Here's how the part is built. I have some questions about the finished solid (model axes, mm). Face numbers are marked on the shaded views. A direction names the side the tool comes from. Give positions to 0.01 mm unless a question says otherwise; leave off trailing zeros. Write each loop counter-clockwise with the first axis right and the second up, starting at its lowest first coordinate (ties: lowest second). Pieces come first, ordered by that corner, then holes. Notation, with made-up numbers: (-38.75, 10.25) - (3.25, 10.25) arc R31 cw to (3.25, 47.25) - close; hole circle Ø4 at (-35.5, 44). An arc over 180 degrees is marked (long way). Use one line per item in the form item = value. Start each with the question number.
from build123d import *

# Parameters (mm, degrees)
SKETCH2_R          = 1.6
CUT_EXTRUDE2_DEPTH = 6
SKETCH4_R          = 1.2
CUT_EXTRUDE4_DEPTH = 5
CHAMFER1_SIZE      = 0.5
CHAMFER3_SIZE      = 0.1


with BuildPart() as part:
    # Sketch1 → Revolve4 (revolve)
    with BuildSketch(Plane.XY, mode=Mode.PRIVATE) as revolve4_sk:
        with BuildLine():
            Line((844.943210176, 281.38888375), (845.428519032, 280.88888375))
            Line((845.428519032, 280.88888375), (849.942387276, 280.88888375))
            Line((849.942387276, 280.88888375), (849.942387276, 290.88888375))
            Line((849.942387276, 290.88888375), (860.942387276, 290.88888375))
            Line((860.942387276, 290.88888375), (860.942387276, 297.88888375))
            Line((860.942387276, 297.88888375), (856.942387276, 297.88888375))
            Line((856.942387276, 297.88888375), (856.942387276, 303.38888375))
            Line((856.942387276, 303.38888375), (853.942387276, 303.38888375))
            Line((853.942387276, 303.38888375), (853.942387276, 302.38888375))
            Line((853.942387276, 302.38888375), (842.942387276, 302.38888375))
            ThreePointArc((842.942387276, 302.38888375), (842.442387276, 302.71356783), (841.942387276, 302.38888375))
            Line((841.942387276, 302.38888375), (840.942387276, 302.38888375))
            Line((840.942387276, 302.38888375), (840.942387276, 299.054998182))
            Line((840.942387276, 299.054998182), (838.850052202, 299.054998182))
            Line((838.850052202, 299.054998182), (838.556543661, 299.38888375))
            Line((838.556543661, 299.38888375), (837.02254839, 299.38888375))
            Line((837.02254839, 299.38888375), (836.904667291, 299.280121777))
            Line((836.904667291, 299.280121777), (836.804319001, 299.38888375))
            Line((836.804319001, 299.38888375), (835.942387276, 299.38888375))
            Line((835.942387276, 299.38888375), (835.942387276, 302.38888375))
            Line((835.942387276, 302.38888375), (834.038239304, 302.38888375))
            Line((834.038239304, 302.38888375), (833.942387276, 302.301556661))
            Line((833.942387276, 302.301556661), (833.862826931, 302.38888375))
            Line((833.862826931, 302.38888375), (831.942387276, 302.38888375))
            Line((831.942387276, 302.38888375), (831.942387276, 261.38888375))
            Line((831.942387276, 261.38888375), (836.942387276, 261.38888375))
            Line((836.942387276, 261.38888375), (836.942387276, 281.38888375))
            Line((836.942387276, 281.38888375), (838.542387276, 281.38888375))
            Line((838.542387276, 281.38888375), (838.791787089, 281.619745582))
            Line((838.791787089, 281.619745582), (843.015951121, 281.619745582))
            Line((843.015951121, 281.619745582), (843.343210176, 281.38888375))
            Line((843.343210176, 281.38888375), (844.943210176, 281.38888375))
        make_face()
    revolve(revolve4_sk.sketch.rotate(Axis((831.942387276, 300.670444461, 0), (0, -1, 0)), 90), axis=Axis((831.942387276, 300.670444461, 0), (0, -1, 0)))

    # Sketch2 → Cut-Extrude2 (cut)
    with BuildSketch(Plane(origin=(0, 302.38888375, 0), x_dir=(-1, 0, 0), z_dir=(0, 1, 0))):
        with Locations(Location((-849.942387276, 0, 0), (0, 0, 90))):
            Circle(SKETCH2_R)
        with Locations(Location((-813.942387276, 0, 0), (0, 0, 90))):
            Circle(SKETCH2_R)
    extrude(amount=-CUT_EXTRUDE2_DEPTH, mode=Mode.SUBTRACT)

    # Cut-Extrude3 cone 1 section (through the dimple's axis) → Cut-Extrude3 (revolve, cut)
    with BuildSketch(Plane(origin=(849.942387276, 296.38888375, 0), x_dir=(0, 0, 1), z_dir=(1, 0, 0))):
        Polygon((0, 0), (1.6, 0), (0, 1.120332061), align=None)
    revolve(axis=Axis((849.942387276, 296.38888375, 0), (0, -1, 0)), mode=Mode.SUBTRACT)

    # Cut-Extrude3 cone 2 section (through the dimple's axis) → Cut-Extrude3 cone 2 (revolve, cut)
    with BuildSketch(Plane(origin=(813.942387276, 296.38888375, 0), x_dir=(0, 0, 1), z_dir=(1, 0, 0))):
        Polygon((0, 0), (1.6, 0), (0, 1.120332061), align=None)
    revolve(axis=Axis((813.942387276, 296.38888375, 0), (0, -1, 0)), mode=Mode.SUBTRACT)

    # Sketch4 → Cut-Extrude4 (cut)
    with BuildSketch(Plane.XZ.offset(-290.88888375)):
        with Locations(Location((831.942387276, -24, 0), (0, 0, 270))):
            Circle(SKETCH4_R)
        with Locations(Location((811.157777585, 12, 0), (0, 0, 270))):
            Circle(SKETCH4_R)
        with Locations(Location((852.726996967, 12, 0), (0, 0, 270))):
            Circle(SKETCH4_R)
    extrude(amount=-CUT_EXTRUDE4_DEPTH, mode=Mode.SUBTRACT)

    # Cut-Extrude5 cone 1 section (through the dimple's axis) → Cut-Extrude5 (revolve, cut)
    with BuildSketch(Plane(origin=(831.942387276, 295.88888375, -24), x_dir=(0, 0, -1), z_dir=(1, 0, 0))):
        Polygon((0, 0), (1.2, 0), (0, 0.840249046), align=None)
    revolve(axis=Axis((831.942387276, 295.88888375, -24), (0, 1, 0)), mode=Mode.SUBTRACT)

    # Cut-Extrude5 cone 2 section (through the dimple's axis) → Cut-Extrude5 cone 2 (revolve, cut)
    with BuildSketch(Plane(origin=(852.726996967, 295.88888375, 12), x_dir=(0, 0, -1), z_dir=(1, 0, 0))):
        Polygon((0, 0), (1.2, 0), (0, 0.840249046), align=None)
    revolve(axis=Axis((852.726996967, 295.88888375, 12), (0, 1, 0)), mode=Mode.SUBTRACT)

    # Cut-Extrude5 cone 3 section (through the dimple's axis) → Cut-Extrude5 cone 3 (revolve, cut)
    with BuildSketch(Plane(origin=(811.157777585, 295.88888375, 12), x_dir=(0, 0, -1), z_dir=(1, 0, 0))):
        Polygon((0, 0), (1.2, 0), (0, 0.840249046), align=None)
    revolve(axis=Axis((811.157777585, 295.88888375, 12), (0, 1, 0)), mode=Mode.SUBTRACT)

    # Chamfer1
    chamfer1_edges = [part.edges().sort_by_distance(p)[0] for p in [
        (831.942387276, 303.38888375, -25),
        (831.942387276, 297.88888375, -29),
        (831.942387276, 290.88888375, -29),
        (831.942387276, 280.88888375, -18),
        (831.942387276, 261.38888375, -5),
        (849.942387276, 302.38888375, -1.6),
        (813.942387276, 302.38888375, -1.6),
        (831.942387276, 290.88888375, -22.8),
        (811.157777585, 290.88888375, 13.2),
        (852.726996967, 290.88888375, 13.2),
    ]]
    chamfer(chamfer1_edges, length=CHAMFER1_SIZE)

    # Chamfer3
    chamfer3_edges = [part.edges().sort_by_distance(p)[0] for p in [
        (831.942387276, 302.38888375, -4),
        (831.942387276, 302.38888375, -9),
        (831.942387276, 303.38888375, -22),
        (831.942387276, 297.88888375, -25),
        (831.942387276, 290.88888375, -18),
    ]]
    chamfer(chamfer3_edges, length=CHAMFER3_SIZE)


solid = part.part
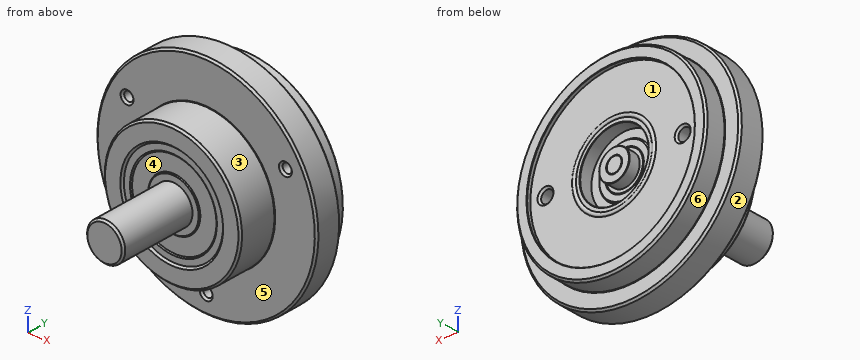
1. We'd pull the mould along Z, two halves only. Please class the marked faces 4, 5 and 6: pulls with the +Z half, pulls with the -Z half, needs draft (parallel to the pull), parting line crosses it, or undercut.
2. For the marked faces 1, 2 and 3, which set-ups out of +Z, -Z, +X, -X, +Y, -Y let a thin tool reach every point of the face, with its end or its side?
3. For P1, Ø3, axis at x = 831.5, z = -1, coming from the +Y side; P2, Ø2, axis at y = 281.5, z = 10, coming from the -X side; P3, Ø20, axis at x = 828.5, z = -1.5, coming from the +Y side; P4, Ø2, axis at x = 820.5, y = 278, coming from the -Z side, each with a flat end and sliding along its axis, tell me the tip position at first contact or that it passes through.
4. I want a section at A-A, the plane y = 267.5. List the corners of the cut face in (x, z) for me, then the cut area to 3 significant figures.
5. Please list where these lines run through material, in increasing order: line 1 (X direction, y = 300, z = 0); line 2 (X direction, y = 299, z = 0); line 3 (Y direction, x = 826.5, z = 7) (3 decimals).
Result sheet:
q1.face_4 = undercut
q1.face_5 = needs draft
q1.face_6 = parting line crosses it
q2.face_1 = +Y
q2.face_2 = +Y, -Y
q2.face_3 = -Y
q3.P1 = 302.39
q3.P2 = 816.35
q3.P3 = 302.71
q3.P4 = through
q4.outline = circle Ø10 at (831.94, 0)
q4.area = 78.5 mm2
q5.line_1 = 806.94 to 812.34, 815.54 to 822.94, 827.94 to 835.94, 840.94 to 848.34, 851.54 to 856.94
q5.line_2 = 806.94 to 812.34, 815.54 to 848.34, 851.54 to 856.94
q5.line_3 = 281.62 to 299.055
